Geometry: final body of the model. Coordinates: model frame, mm. Face numbers are marked on the shaded views. A direction names the side the tool comes from. Coordinates: 2 decimals unless noted, no trailing zeros. Order: outer loops, then holes, each group sorted by start corner. A loop starts at its lowest first (then second) coordinate and runs counter-clockwise, first axis right, second up. Notation, with made-up numbers: M -17,-33.75 L 4,-33.75 A10 cw 4,-16.75 Z; hole C 79,33 d6. An arc over 180 degrees is marked long. One line per question, with ' | ' between items.
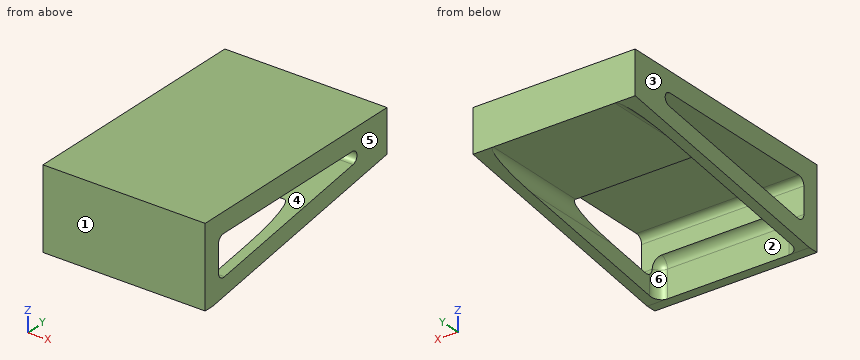
from build123d import *

# Parameters (mm, degrees)
SKETCH1_W                       = 152.4
SKETCH1_H                       = 40
BOSS_EXTRUDE1_DEPTH             = 179.05
BOSS_EXTRUDE1_DEPTH_BACK        = 100
BOSS_EXTRUDE2_REACH             = 200.659
SKETCH3_W                       = 75
SKETCH3_H                       = 9.525
BOSS_EXTRUDE2_DIRECTION_2_REACH = 200.659
RIB1_REACH                      = 248.799
SKETCH4_WALL_W                  = 715.816770022
SKETCH4_WALL_H                  = 9.525
FILLET1_R                       = 9.525
CUT_EXTRUDE1_REACH              = 210.543
CUT_EXTRUDE1_DIRECTION_2_REACH  = 210.543


with BuildPart() as part:
    # Sketch1 → Boss-Extrude1 (new, two sides)
    with BuildSketch(Plane(origin=(0, 0, 0), x_dir=(1, 0, 0), z_dir=(0, 1, 0))) as boss_extrude1_sk:
        with Locations((0, 20)):
            Rectangle(SKETCH1_W, SKETCH1_H)
    extrude(amount=BOSS_EXTRUDE1_DEPTH)
    extrude(boss_extrude1_sk.sketch, amount=-BOSS_EXTRUDE1_DEPTH_BACK)

    # SurfaceCut1
    split(bisect_by=Plane(origin=(0, -47.895, 0), x_dir=(1, 0, 0), z_dir=(0, 1, 0)), keep=Keep.TOP)

    # Boss-Extrude2: up to this face of the body (flat: up to its plane)
    boss_extrude2_end = Plane(part.part.faces().sort_by_distance((76.2, 65.5775, -20))[0])
    # Sketch3 → Boss-Extrude2 (add, up to the picked face)
    with BuildSketch(Plane(origin=(0, 0, 0), x_dir=(0, 0, -1), z_dir=(1, 0, 0)), mode=Mode.PRIVATE) as boss_extrude2_sk1:
        with Locations((37.5, -43.1325)):
            Rectangle(SKETCH3_W, SKETCH3_H)
    boss_extrude2_tool1 = split(extrude(boss_extrude2_sk1.sketch, amount=BOSS_EXTRUDE2_REACH, mode=Mode.PRIVATE), bisect_by=boss_extrude2_end, keep=Keep.BOTH, mode=Mode.PRIVATE)
    add(boss_extrude2_tool1.solids().sort_by(Axis((0, -43.1325, -37.5), (1, 0, 0)))[0])

    # Boss-Extrude2 direction 2: up to this face of the body (flat: up to its plane)
    boss_extrude2_direction_2_end = Plane(part.part.faces().sort_by_distance((-76.2, 65.5775, -20))[0])
    # Sketch3 → Boss-Extrude2 direction 2 (add, up to the picked face)
    with BuildSketch(Plane(origin=(0, 0, 0), x_dir=(0, 0, -1), z_dir=(1, 0, 0)), mode=Mode.PRIVATE) as boss_extrude2_direction_2_sk1:
        with Locations((37.5, -43.1325)):
            Rectangle(SKETCH3_W, SKETCH3_H)
    boss_extrude2_direction_2_tool1 = split(extrude(boss_extrude2_direction_2_sk1.sketch, amount=-BOSS_EXTRUDE2_DIRECTION_2_REACH, mode=Mode.PRIVATE), bisect_by=boss_extrude2_direction_2_end, keep=Keep.BOTH, mode=Mode.PRIVATE)
    add(boss_extrude2_direction_2_tool1.solids().sort_by(Axis((0, -43.1325, -37.5), (-1, 0, 0)))[0])

    # Sketch4 wall → Rib1 (add, up to next)
    with BuildSketch(Plane(origin=(76.2, 70.34, -57.5), x_dir=(0, -0.987289431969, -0.158932619441), z_dir=(0, 0.158932619441, -0.987289431969)), mode=Mode.PRIVATE) as rib1_sk1:
        with Locations((0, 4.7625)):
            Rectangle(SKETCH4_WALL_W, SKETCH4_WALL_H)
    rib1_tool1 = extrude(rib1_sk1.sketch, amount=-RIB1_REACH, mode=Mode.PRIVATE) - part.part
    rib1 = rib1_tool1.solids().sort_by_distance((76.2, 70.34, -57.5))[0]
    add(rib1)

    # Mirror1: Rib1 across plane
    add(rib1.mirror(Plane(origin=(0, 0, 0), x_dir=(0, 0, 1), z_dir=(1, 0, 0))))

    # Fillet1
    fillet1_edges = [part.edges().sort_by_distance(p)[0] for p in [
        (0, -38.37, -40),
        (66.675, -38.37, -57.5),
        (66.675, 70.34, -40),
        (-66.675, 70.34, -40),
        (-66.675, -38.37, -57.5),
    ]]
    fillet(fillet1_edges, radius=FILLET1_R)

    # Cut-Extrude1: up to this face of the body (flat: up to its plane)
    cut_extrude1_end = Plane(part.part.faces().sort_by_distance((-76.2, 53.773975166, -30.062668553))[0])
    # Sketch8 → Cut-Extrude1 (cut, up to the picked face)
    with BuildSketch(Plane(origin=(0, 0, 0), x_dir=(0, 0, -1), z_dir=(1, 0, 0)), mode=Mode.PRIVATE) as cut_extrude1_sk1:
        with BuildLine():
            Line((25.236746286, -31.487519231), (49.576175238, -31.487519231))
            ThreePointArc((49.576175238, -31.487519231), (54.633662665, -29.152106057), (56.135591687, -23.787728834))
            Line((56.135591687, -23.787728834), (30.301291161, 136.694946031))
            ThreePointArc((30.301291161, 136.694946031), (24.071010718, 141.587364194), (18.697485511, 135.766936654))
            Line((18.697485511, 135.766936654), (18.697485511, -24.948258456))
            ThreePointArc((18.697485511, -24.948258456), (20.612790648, -29.572214094), (25.236746286, -31.487519231))
        make_face()
    cut_extrude1_tool1 = split(extrude(cut_extrude1_sk1.sketch, amount=-CUT_EXTRUDE1_REACH, mode=Mode.PRIVATE), bisect_by=cut_extrude1_end, keep=Keep.BOTH, mode=Mode.PRIVATE)
    add(cut_extrude1_tool1.solids().sort_by(Axis((0, 38.89099, -32.356169), (-1, 0, 0)))[0], mode=Mode.SUBTRACT)

    # Cut-Extrude1 direction 2: up to this face of the body (flat: up to its plane)
    cut_extrude1_direction_2_end = Plane(part.part.faces().sort_by_distance((76.2, 53.773975166, -30.062668553))[0])
    # Sketch8 → Cut-Extrude1 direction 2 (cut, up to the picked face)
    with BuildSketch(Plane(origin=(0, 0, 0), x_dir=(0, 0, -1), z_dir=(1, 0, 0)), mode=Mode.PRIVATE) as cut_extrude1_direction_2_sk1:
        with BuildLine():
            Line((25.236746286, -31.487519231), (49.576175238, -31.487519231))
            ThreePointArc((49.576175238, -31.487519231), (54.633662665, -29.152106057), (56.135591687, -23.787728834))
            Line((56.135591687, -23.787728834), (30.301291161, 136.694946031))
            ThreePointArc((30.301291161, 136.694946031), (24.071010718, 141.587364194), (18.697485511, 135.766936654))
            Line((18.697485511, 135.766936654), (18.697485511, -24.948258456))
            ThreePointArc((18.697485511, -24.948258456), (20.612790648, -29.572214094), (25.236746286, -31.487519231))
        make_face()
    cut_extrude1_direction_2_tool1 = split(extrude(cut_extrude1_direction_2_sk1.sketch, amount=CUT_EXTRUDE1_DIRECTION_2_REACH, mode=Mode.PRIVATE), bisect_by=cut_extrude1_direction_2_end, keep=Keep.BOTH, mode=Mode.PRIVATE)
    add(cut_extrude1_direction_2_tool1.solids().sort_by(Axis((0, 38.89099, -32.356169), (1, 0, 0)))[0], mode=Mode.SUBTRACT)


solid = part.part
1. Material intervals for line 1 (X direction, y = -25.5, z = -68) (3 decimals); line 2 (Z direction, x = -25, y = 14); line 3 (Z direction, x = 1, y = 141), sorted ascending. Write a range as [from, to].
Response values:
line 1: x = [-76.2, -66.675], [66.675, 76.2] | line 2: z = [-18.7, 0] | line 3: z = [-40, -27.13], [-21.95, 0]
2. Section A-A, the plane y = 46. Output: boundary loops of the cut face in (x, z) (3 decimals).
Response values:
outline: M -76.2,-61.418 L -66.675,-61.418 L -66.675,-49.525 A9.525 cw -65.477,-44.901 L -76.2,-44.901 Z; M -76.2,-18.697 L 76.2,-18.697 L 76.2,0 L -76.2,0 Z; M 65.477,-44.901 A9.525 cw 66.675,-49.525 L 66.675,-61.418 L 76.2,-61.418 L 76.2,-44.901 Z
3. Draft query along X for the marked faces 1, 2 and 3. Return one class per face: pulls with the +X half, pulls with the -X half, needs draft (parallel to the pull), parting line crosses it, or undercut.
Response values:
face 1: needs draft | face 2: undercut | face 3: pulls with the -X half
4. Access query for the marked faces 4, 5 and 6. Directions: +Z, -Z, +X, -X, +Y, -Y. A direction counts if a zero-diameter tool reaches every point of the face in a straight line with its end or side. Return the directions, or none.
Response values:
face 4: +X, -X | face 5: +Z, -Z, +X, +Y, -Y | face 6: -Z, +Y
5. Pin query (flat end, axial travel): P1, Ø19, axis at y = 81.5, z = -64, coming from the -X side; P2, Ø12.5, axis at x = 26.5, z = -66.5, coming from the +Y side; P3, Ø1.5, axis at x = -43, y = 37, coming from the -Z side; P4, Ø8, axis at x = -30, z = -47.5, coming from the +Y side. Return the tip coordinate at first contact, or that it passes through.
Response values:
P1: stops at x = -76.2 | P2: stops at y = -38.37 | P3: stops at z = -18.7 | P4: stops at y = -36.22
6. Section D-D, the plane y = 116.5. Output: boundary loops of the cut face in (x, z) (3 decimals).
Response values:
outline: M -76.2,-50.069 L -66.675,-50.069 L -66.675,-49.525 A9.525 cw -57.15,-40 L 57.15,-40 A9.525 cw 66.675,-49.525 L 66.675,-50.069 L 76.2,-50.069 L 76.2,-33.552 L -76.2,-33.552 Z; M -76.2,-18.697 L 76.2,-18.697 L 76.2,0 L -76.2,0 Z
7. Section B-B, the plane z = -34.5. Output: boundary loops of the cut face in (x, y) (3 decimals), and give its area (3 significant figures).
Response values:
outline: M -76.2,-47.895 L 76.2,-47.895 L 76.2,-31.488 L -76.2,-31.488 Z; M -76.2,110.613 L 76.2,110.613 L 76.2,179.05 L -76.2,179.05 Z | area: 12,900 mm^2
